from build123d import *

# Parameters (mm, degrees)
SKETCH2_R           = 115
SKETCH2_R_2         = 105
BOSS_EXTRUDE1_DEPTH = 260
CUT_EXTRUDE1_REACH  = 117
SKETCH3_W           = 2
SKETCH3_H           = 15


with BuildPart() as part:
    # Sketch2 → Boss-Extrude1 (new body)
    with BuildSketch(Plane.XY):
        Circle(SKETCH2_R)
        Circle(SKETCH2_R_2, mode=Mode.SUBTRACT)
    extrude(amount=BOSS_EXTRUDE1_DEPTH)

    # Sketch3 → Cut-Extrude1 (cut, up to next)
    with BuildSketch(Plane(origin=(0, 0, 0), x_dir=(0, 0, -1), z_dir=(1, 0, 0)), mode=Mode.PRIVATE) as cut_extrude1_sk1:
        with Locations((-1, 0)):
            Rectangle(SKETCH3_W, SKETCH3_H)
    cut_extrude1_tool1 = extrude(cut_extrude1_sk1.sketch, amount=-CUT_EXTRUDE1_REACH, mode=Mode.PRIVATE) & part.part
    add(cut_extrude1_tool1.solids().sort_by_distance((0, 0, 1))[0], mode=Mode.SUBTRACT)


solid = part.part
Part model, mm, in its own coordinate system. Round coordinates to 2 decimals unless told otherwise and drop trailing zeros. Write each loop counter-clockwise with the first axis right and the second up, starting at its lowest first coordinate (ties: lowest second). Pieces come first, ordered by that corner, then holes. Notation, with made-up numbers: M 10.25,83 L 46.25,83 A29 cw 46.25,107 Z; hole C 38,12 d6. An arc over 180 degrees is marked long. Return JSON: item names as keys, results as strings. Group by question number.
(1) Saw through at A-A on x = 0. Write the cut outline in (y, z), then the cut area to 3 significant figures.
(2) Saw through at C-C on z = 175. Write the cut outline in (x, y), then the cut area to 3 significant figures.
(3) Pin check, flat tips, straight feed: pin 1 Ø12 at (x, z) = (69.5, 102.5) entering from +Y; pin 2 Ø6 at (y, z) = (-87, 30.5) entering from -X; pin 3 Ø8 at (x, z) = (-49, 142.5) entering from -Y. Stop position of each tip, or through.
(4) Saw through at B-B on y = 0. Write the cut outline in (x, z).
(5) Two-plate mould, pull along X, no slides. Class faces 1 (the face through (-24.93, -112.265, 128.18)), 2 (the face through (-110, 0, 2)), 3 (the face through (100.15, 31.54, 128.18)): +X half, -X half, draft (parallel to the pull), parting line (faces both ways), or undercut.
(6) Drill centre lines: probe 1 along Y at (x, z) = (0, 128); probe 2 along Y at (x, z) = (62, 115). Where is each one in solid material? Low to high.
Returned:
{
 "1": {"outline": "M -115,0 L -105,0 L -105,260 L -115,260 Z; M 105,0 L 115,0 L 115,260 L 105,260 Z", "area": "5,200 mm²"},
 "2": {"outline": "C 0,0 d230; hole C 0,0 d210", "area": "6,910 mm²"},
 "3": {"pin 1": "y = 95.88", "pin 2": "x = -78.54", "pin 3": "y = -105.83"},
 "4": {"outline": "M -115,2 L -105,2 L -105,260 L -115,260 Z; M 105,0 L 115,0 L 115,260 L 105,260 Z"},
 "5": {"face 1": "parting line", "face 2": "draft", "face 3": "undercut"},
 "6": {"probe 1": "-115 to -105, 105 to 115", "probe 2": "-96.86 to -84.74, 84.74 to 96.86"}
}
